Here's how the part is built. I have some questions about the finished solid (model axes, mm). A direction names the side the tool comes from. Coordinates: 2 decimals unless noted, no trailing zeros. Write each loop counter-clockwise with the first axis right and the second up, starting at its lowest first coordinate (ties: lowest second). Pieces come first, ordered by that corner, then holes. Notation, with made-up numbers: M 23.25,-8.5 L 60.25,-8.5 A26 ccw 60.25,21.5 Z; hole C 23.25,79 d6. An arc over 180 degrees is marked long. Use a Markdown table: item, result.
```python
from build123d import *

# Parameters (mm, degrees)
BOSS_EXTRUDE1_DEPTH = 10
FILLET1_R           = 2
FILLET2_R           = 2
FILLET3_R           = 2
FILLET4_R           = 2
FILLET5_R           = 1
FILLET6_R           = 2
FILLET7_R           = 1


with BuildPart() as part:
    # Sketch1 → Boss-Extrude1 (new body)
    with BuildSketch(Plane(origin=(0, 0, 0), x_dir=(1, 0, 0), z_dir=(0, 1, 0))):
        Polygon((0, 0), (0, 6), (2.1, 6), (2.1, -26), (-17.9, -26), (-17.9, -29), (5.1, -29), (5.1, 9), (-3, 9), (-3, 0), align=None)
    extrude(amount=BOSS_EXTRUDE1_DEPTH)

    # Fillet1
    fillet1_edges = [part.edges().sort_by_distance(p)[0] for p in [
        (5.1, 5, -9),
    ]]
    fillet(fillet1_edges, radius=FILLET1_R)

    # Fillet2
    fillet2_edges = [part.edges().sort_by_distance(p)[0] for p in [
        (5.1, 5, 29),
    ]]
    fillet(fillet2_edges, radius=FILLET2_R)

    # Fillet3
    fillet3_edges = [part.edges().sort_by_distance(p)[0] for p in [
        (-17.9, 5, 29),
    ]]
    fillet(fillet3_edges, radius=FILLET3_R)

    # Fillet4
    fillet4_edges = [part.edges().sort_by_distance(p)[0] for p in [
        (-3, 5, -9),
    ]]
    fillet(fillet4_edges, radius=FILLET4_R)

    # Fillet5
    fillet5_edges = [part.edges().sort_by_distance(p)[0] for p in [
        (-17.9, 5, 26),
    ]]
    fillet(fillet5_edges, radius=FILLET5_R - 0.0001)  # a hair under: the kernel refuses the full size

    # Fillet6
    fillet6_edges = [part.edges().sort_by_distance(p)[0] for p in [
        (-3, 5, 0),
    ]]
    fillet(fillet6_edges, radius=FILLET6_R)

    # Fillet7
    fillet7_edges = [part.edges().sort_by_distance(p)[0] for p in [
        (0, 5, 0),
    ]]
    fillet(fillet7_edges, radius=FILLET7_R - 0.0001)  # a hair under: the kernel refuses the full size


solid = part.part
```
1. Suppose I cut it at D-D on x = -8. Write out the boundary of the cut face in (y, z).
Answers follow:
| item | result |
|---|---|
| outline | M 0,26 L 10,26 L 10,29 L 0,29 Z |
2. I need wall thicknesses on probe 1 along X at (y, z) = (3, -3); probe 2 along X at (y, z) = (8.5, 9); probe 3 along Z at (x, y) = (-8.5, 1). Which ranges of each line are inside material? Lowest first, please.
Answers follow:
| item | result |
|---|---|
| probe 1 | x = -3 to 0, 2.1 to 5.1 |
| probe 2 | x = 2.1 to 5.1 |
| probe 3 | z = 26 to 29 |
3. Will these pins go through, and if not, where does the flat tip stop? pin 1 Ø2 at (x, y) = (-3.5, 5.5) entering from -Z; pin 2 Ø5 at (y, z) = (3, 6) entering from -X; pin 3 Ø6 at (x, y) = (-11.5, 7) entering from -Z; pin 4 Ø8 at (x, z) = (2, -3.5) entering from -Y.
Answers follow:
| item | result |
|---|---|
| pin 1 | stops at z = -8.32 |
| pin 2 | stops at x = 2.1 |
| pin 3 | stops at z = 26 |
| pin 4 | stops at y = 0 |
4. Which directions (+Z, -Z, +X, -X, +Y, -Y) give clear straight access to the entire face, cutting with the end or side of a thin tool? Please do faces 1 (the face through (-3, 5, -5)), 2 (the face through (2.1, 5, 10)), 3 (the face through (-7, 5, 26)).
Answers follow:
| item | result |
|---|---|
| face 1 | -Z, -X, +Y, -Y |
| face 2 | +Y, -Y |
| face 3 | -X, +Y, -Y |
5. Suppose I cut it at C-C on z = 3. Write out the boundary of the cut face in (x, y).
Answers follow:
| item | result |
|---|---|
| outline | M 2.1,0 L 5.1,0 L 5.1,10 L 2.1,10 Z |
6. Suppose I cut it at A-A on x = 1.25. Write out the boundary of the cut face in (y, z), and give its area (3 significant figures).
Answers follow:
| item | result |
|---|---|
| outline | M 0,-9 L 10,-9 L 10,-6 L 0,-6 Z; M 0,26 L 10,26 L 10,29 L 0,29 Z |
| area | 60.0 mm2 |
7. We'd pull the mould along Z, two halves only. Please class faces 4 (the face through (-7, 5, 29)), 5 (the face through (-17.615, 5.07, 26.301)), 6 (the face through (0, 5, -3)), 7 (the face through (5.1, 5, 10)): +Z half, -Z half, draft (parallel to the pull), parting line (faces both ways), or undercut.
Answers follow:
| item | result |
|---|---|
| face 4 | +Z half |
| face 5 | -Z half |
| face 6 | undercut |
| face 7 | draft |
